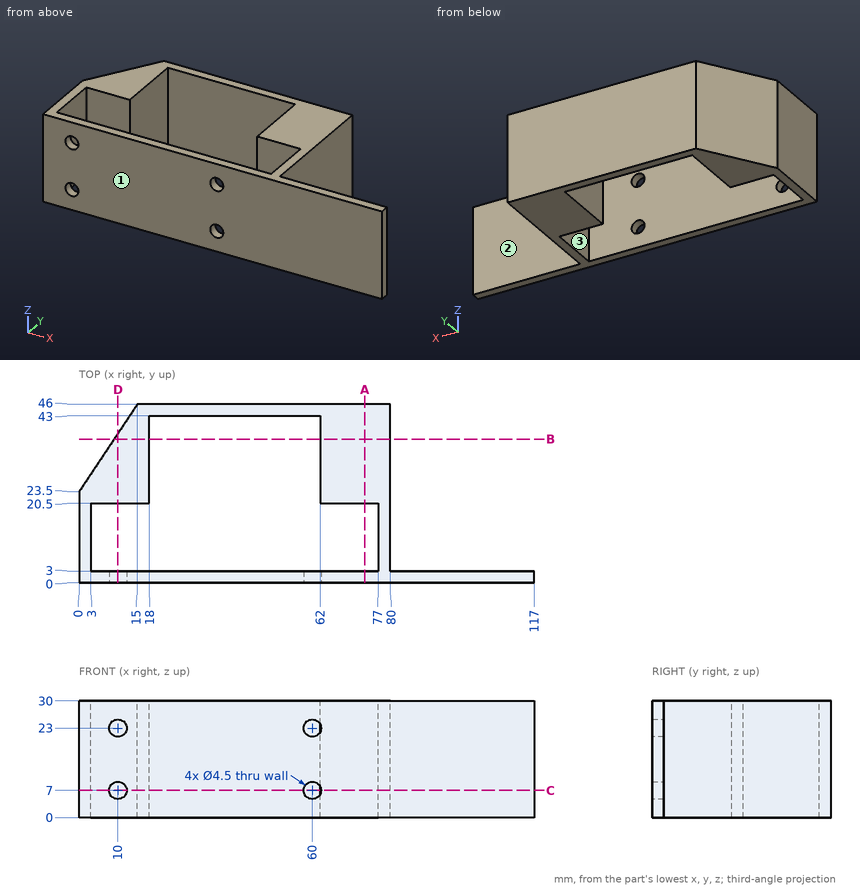
Source: three-view drawing plus pictorial views. Frame: mm from the lowest corner of the part. A direction names the side the tool comes from. Round coordinates to 2 decimals unless told otherwise and drop trailing zeros. Write each loop counter-clockwise with the first axis right and the second up, starting at its lowest first coordinate (ties: lowest second). Pieces come first, ordered by that corner, then holes. Notation, with made-up numbers: (81.25, 48.5) -> (128.25, 48.5) arc R32 ccw to (128.25, 86.5) -> close; hole circle Ø6 at (-40, 26). An arc over 180 degrees is marked (long way). Return JSON: item names as keys, results as strings.
Q1. Ray query, line 1 (X direction, y = 1.1, z = 23); line 2 (X direction, y = 19, z = 4.5); line 3 (Y direction, x = 73, z = 13). Return the intervals inside material, ascending.
From the geometry:
{"line 1": "0 to 7.75, 12.25 to 57.75, 62.25 to 117", "line 2": "0 to 3, 77 to 80", "line 3": "0 to 3, 20.5 to 46"}
Q2. Section C-C on z = 7. Return the cut outline in (x, y).
From the geometry:
{"outline": "(0, 0) -> (7.75, 0) -> (7.75, 3) -> (3, 3) -> (3, 20.5) -> (18, 20.5) -> (18, 43) -> (62, 43) -> (62, 20.5) -> (77, 20.5) -> (77, 3) -> (62.25, 3) -> (62.25, 0) -> (117, 0) -> (117, 3) -> (80, 3) -> (80, 46) -> (15, 46) -> (0, 23.5) -> close; (12.25, 0) -> (57.75, 0) -> (57.75, 3) -> (12.25, 3) -> close"}
Q3. Set-up query: the marked faces 1, 2 and 3. Return all of +Z, -Z, +X, -X, +Y, -Y with unobstructed straight access to the full face (end or side cutting, diameter ignored); none if empty.
From the geometry:
{"face 1": "+Z, -Z, +X, -X, -Y", "face 2": "+Z, -Z, +X, +Y", "face 3": "+Z, -Z"}
Q4. Section A-A on x = 73.5. Return the cut outline in (y, z), and give its area (3 significant figures).
From the geometry:
{"outline": "(0, 0) -> (3, 0) -> (3, 30) -> (0, 30) -> close; (20.5, 0) -> (46, 0) -> (46, 30) -> (20.5, 30) -> close", "area": "855 mm2"}
Q5. Section B-B on y = 37. Return the cut outline in (x, z).
From the geometry:
{"outline": "(9, 0) -> (18, 0) -> (18, 30) -> (9, 30) -> close; (62, 0) -> (80, 0) -> (80, 30) -> (62, 30) -> close"}
Q6. Section D-D on x = 10. Return the cut outline in (y, z).
From the geometry:
{"outline": "(0, 0) -> (3, 0) -> (3, 4.75) -> (0, 4.75) -> close; (0, 9.25) -> (3, 9.25) -> (3, 20.75) -> (0, 20.75) -> close; (0, 25.25) -> (3, 25.25) -> (3, 30) -> (0, 30) -> close; (20.5, 0) -> (38.5, 0) -> (38.5, 30) -> (20.5, 30) -> close"}
Q7. First-contact query: pin 1 Ø6 at (x, z) = (10, 7) entering from +Y; pin 2 Ø4 at (y, z) = (38.5, 7.5) entering from +X; pin 3 Ø1.5 at (x, y) = (19.5, 33.5) entering from -Z. Flat tips, straight axial feed; report the tip coordinate or a pass-through.
From the geometry:
{"pin 1": "y = 43", "pin 2": "x = 80", "pin 3": "through"}
